from build123d import *

# Parameters (mm, degrees)
SKETCH_1_R          = 9.9
SKETCH_1_R_2        = 1.85
EXTRUDE_1_DEPTH     = 7
SKETCH_2_R          = 12.5
SKETCH_2_R_2        = 1.85
EXTRUDE_2_DEPTH     = 2.5
SKETCH_3_R          = 3.75
EXTRUDE_3_DEPTH     = 6.3
CHAMFER_1_SIZE      = 2
SKETCH_4_R          = 41.5
CUT_EXTRUDE_1_DEPTH = 15.5
EXTRUDE_START       = -0.3
SKETCH_5_R          = 12
SKETCH_5_R_2        = 9.9
EXTRUDE_4_DEPTH     = 0.3


with BuildPart() as part:
    # 草图1 → 凸台-拉伸1 (new body)
    with BuildSketch(Plane(origin=(0, 0, 0), x_dir=(1, 0, 0), z_dir=(0, 1, 0))):
        with Locations(Location((0, 0, 0), (0, 0, 270))):
            Circle(SKETCH_1_R)
        with Locations(Location((6, 0, 0), (0, 0, 270))):
            Circle(SKETCH_1_R_2, mode=Mode.SUBTRACT)
        with Locations(Location((0, -6, 0), (0, 0, 270))):
            Circle(SKETCH_1_R_2, mode=Mode.SUBTRACT)
        with Locations(Location((-6, 0, 0), (0, 0, 270))):
            Circle(SKETCH_1_R_2, mode=Mode.SUBTRACT)
        with Locations(Location((0, 6, 0), (0, 0, 270))):
            Circle(SKETCH_1_R_2, mode=Mode.SUBTRACT)
    extrude(amount=EXTRUDE_1_DEPTH)

    # 草图2 → 凸台-拉伸2 (add)
    with BuildSketch(Plane(origin=(0, 7, 0), x_dir=(1, 0, 0), z_dir=(0, 1, 0))):
        with Locations(Location((0, 0, 0), (0, 0, 270))):
            Circle(SKETCH_2_R)
        with Locations(Location((-6, 0, 0), (0, 0, 270))):
            Circle(SKETCH_2_R_2, mode=Mode.SUBTRACT)
        with Locations(Location((0, -6, 0), (0, 0, 270))):
            Circle(SKETCH_2_R_2, mode=Mode.SUBTRACT)
        with Locations(Location((6, 0, 0), (0, 0, 270))):
            Circle(SKETCH_2_R_2, mode=Mode.SUBTRACT)
        with Locations(Location((0, 6, 0), (0, 0, 270))):
            Circle(SKETCH_2_R_2, mode=Mode.SUBTRACT)
    extrude(amount=EXTRUDE_2_DEPTH)

    # 草图3 → 凸台-拉伸3 (add)
    # profile 1 of 8: a face of its own
    with BuildSketch(Plane(origin=(0, 9.5, 0), x_dir=(1, 0, 0), z_dir=(0, 1, 0))):
        with BuildLine():
            Line((2.25, 0), (-2.25, 0))
            ThreePointArc((-2.25, 0), (-6, -3.75), (-9.75, 0))
            Line((-9.75, 0), (-12.5, 0))
            ThreePointArc((-12.5, 0), (-3.952847075, -11.858541226), (10, -7.5))
            ThreePointArc((10, -7.5), (11.858541226, -3.952847075), (12.5, 0))
            Line((12.5, 0), (9.75, 0))
            ThreePointArc((9.75, 0), (6, -3.75), (2.25, 0))
        make_face()
        with Locations(Location((0, -6, 0), (0, 0, 270))):
            Circle(SKETCH_3_R, mode=Mode.SUBTRACT)
    # profile 2 of 8: a face of its own
    with BuildSketch(Plane(origin=(0, 9.5, 0), x_dir=(1, 0, 0), z_dir=(0, 1, 0))):
        with BuildLine():
            ThreePointArc((-9.75, 0), (-6, 3.75), (-2.25, 0))
            Line((-2.25, 0), (2.25, 0))
            ThreePointArc((2.25, 0), (6, 3.75), (9.75, 0))
            Line((9.75, 0), (12.5, 0))
            ThreePointArc((12.5, 0), (11.858541226, 3.952847075), (10, 7.5))
            ThreePointArc((10, 7.5), (-3.952847075, 11.858541226), (-12.5, 0))
            Line((-12.5, 0), (-9.75, 0))
        make_face()
        with Locations(Location((0, 6, 0), (0, 0, 270))):
            Circle(SKETCH_3_R, mode=Mode.SUBTRACT)
    # profile 3 of 8: a face of its own
    with BuildSketch(Plane(origin=(0, 9.5, 0), x_dir=(1, 0, 0), z_dir=(0, 1, 0))):
        with BuildLine():
            ThreePointArc((10, 7.5), (11.858541226, 3.952847075), (12.5, 0))
            Line((12.5, 0), (25.5, 0))
            ThreePointArc((25.5, 0), (27.696699141, 5.303300859), (33, 7.5))
            Line((33, 7.5), (10, 7.5))
        make_face()
    # profile 4 of 8: a face of its own
    with BuildSketch(Plane(origin=(0, 9.5, 0), x_dir=(1, 0, 0), z_dir=(0, 1, 0))):
        with BuildLine():
            Line((25.5, 0), (12.5, 0))
            ThreePointArc((12.5, 0), (11.858541226, -3.952847075), (10, -7.5))
            Line((10, -7.5), (33, -7.5))
            ThreePointArc((33, -7.5), (27.696699141, -5.303300859), (25.5, 0))
        make_face()
    # profile 5 of 8: a face of its own
    with BuildSketch(Plane(origin=(0, 9.5, 0), x_dir=(1, 0, 0), z_dir=(0, 1, 0))):
        with BuildLine():
            ThreePointArc((33, 7.5), (27.696699141, 5.303300859), (25.5, 0))
            Line((25.5, 0), (28.65, 0))
            ThreePointArc((28.65, 0), (33, 4.35), (37.35, 0))
            Line((37.35, 0), (40.5, 0))
            ThreePointArc((40.5, 0), (38.303300859, 5.303300859), (33, 7.5))
        make_face()
    # profile 6 of 8: a face of its own
    with BuildSketch(Plane(origin=(0, 9.5, 0), x_dir=(1, 0, 0), z_dir=(0, 1, 0))):
        with BuildLine():
            Line((28.65, 0), (25.5, 0))
            ThreePointArc((25.5, 0), (27.696699141, -5.303300859), (33, -7.5))
            ThreePointArc((33, -7.5), (38.303300859, -5.303300859), (40.5, 0))
            Line((40.5, 0), (37.35, 0))
            ThreePointArc((37.35, 0), (33, -4.35), (28.65, 0))
        make_face()
    # profile 7 of 8: a face of its own
    with BuildSketch(Plane(origin=(0, 9.5, 0), x_dir=(1, 0, 0), z_dir=(0, 1, 0))):
        with BuildLine():
            ThreePointArc((33, 7.5), (27.696699141, 5.303300859), (25.5, 0))
            Line((25.5, 0), (28.65, 0))
            ThreePointArc((28.65, 0), (33, 4.35), (37.35, 0))
            Line((37.35, 0), (40.5, 0))
            ThreePointArc((40.5, 0), (38.303300859, 5.303300859), (33, 7.5))
        make_face()
    # profile 8 of 8: a face of its own
    with BuildSketch(Plane(origin=(0, 9.5, 0), x_dir=(1, 0, 0), z_dir=(0, 1, 0))):
        with BuildLine():
            Line((28.65, 0), (25.5, 0))
            ThreePointArc((25.5, 0), (27.696699141, -5.303300859), (33, -7.5))
            ThreePointArc((33, -7.5), (38.303300859, -5.303300859), (40.5, 0))
            Line((40.5, 0), (37.35, 0))
            ThreePointArc((37.35, 0), (33, -4.35), (28.65, 0))
        make_face()
    extrude(amount=EXTRUDE_3_DEPTH)

    # 倒角1
    # the kernel refuses this chamfer: 2 mm, written as the material it adds along each edge
    with BuildSketch(Plane(origin=(0, 9.5, 6), x_dir=(0, 0, 1), z_dir=(-1, 0, 0))) as chamfer_1_piece_1_section:
        Polygon((3.75 - CHAMFER_1_SIZE, 0), (3.75, CHAMFER_1_SIZE), (3.75, 0), align=None)
    chamfer_1_piece_1 = revolve(axis=Axis((0, 9.5, 6), (0, 1, 0)), mode=Mode.PRIVATE)
    chamfer_1_piece_1 = chamfer_1_piece_1 - Plane(origin=(0, 10.553600351, 6), x_dir=(0, 0, 1), z_dir=(0, -1, 0)) * Cylinder(1.85, 15, mode=Mode.PRIVATE)
    add(chamfer_1_piece_1)
    with BuildSketch(Plane(origin=(-6, 9.5, 0), x_dir=(-1, 0, 0), z_dir=(0, 0, 1))) as chamfer_1_piece_2_section:
        Polygon((3.75 - CHAMFER_1_SIZE, 0), (3.75, -CHAMFER_1_SIZE), (3.75, 0), align=None)
    chamfer_1_piece_2 = revolve(axis=Axis((-6, 9.5, 0), (0, -1, 0)), mode=Mode.PRIVATE)
    chamfer_1_piece_2 = chamfer_1_piece_2 - Plane(origin=(-6, 10.553600351, 0), x_dir=(0, 0, 1), z_dir=(0, -1, 0)) * Cylinder(1.85, 15, mode=Mode.PRIVATE)
    add(chamfer_1_piece_2)
    with BuildSketch(Plane(origin=(0, 9.5, -6), x_dir=(0, 0, 1), z_dir=(-1, 0, 0))) as chamfer_1_piece_3_section:
        Polygon((3.75 - CHAMFER_1_SIZE, 0), (3.75, CHAMFER_1_SIZE), (3.75, 0), align=None)
    chamfer_1_piece_3 = revolve(axis=Axis((0, 9.5, -6), (0, 1, 0)), mode=Mode.PRIVATE)
    chamfer_1_piece_3 = chamfer_1_piece_3 - Plane(origin=(0, 10.553600351, -6), x_dir=(0, 0, 1), z_dir=(0, -1, 0)) * Cylinder(1.85, 16, mode=Mode.PRIVATE)
    add(chamfer_1_piece_3)
    with BuildSketch(Plane(origin=(6, 9.5, 0), x_dir=(1, 0, 0), z_dir=(0, 0, -1))) as chamfer_1_piece_4_section:
        Polygon((3.75 - CHAMFER_1_SIZE, 0), (3.75, -CHAMFER_1_SIZE), (3.75, 0), align=None)
    chamfer_1_piece_4 = revolve(axis=Axis((6, 9.5, 0), (0, -1, 0)), mode=Mode.PRIVATE)
    chamfer_1_piece_4 = chamfer_1_piece_4 - Plane(origin=(6, 10.553600351, 0), x_dir=(0, 0, 1), z_dir=(0, -1, 0)) * Cylinder(1.85, 15, mode=Mode.PRIVATE)
    add(chamfer_1_piece_4)

    # 草图4 → 切除-拉伸1 (cut)
    with BuildSketch(Plane(origin=(0, 15.8, 0), x_dir=(1, 0, 0), z_dir=(0, 1, 0))):
        Circle(SKETCH_4_R)
    extrude(amount=-CUT_EXTRUDE_1_DEPTH, mode=Mode.SUBTRACT)

    # 草图5 → 凸台-拉伸4 (add)
    with BuildSketch(Plane(origin=(0, 0.3, 0), x_dir=(1, 0, 0), z_dir=(0, 1, 0)).offset(EXTRUDE_START)):
        with Locations(Location((0, 0, 0), (0, 0, 270))):
            Circle(SKETCH_5_R)
        Circle(SKETCH_5_R_2, mode=Mode.SUBTRACT)
    extrude(amount=EXTRUDE_4_DEPTH)


solid = part.part
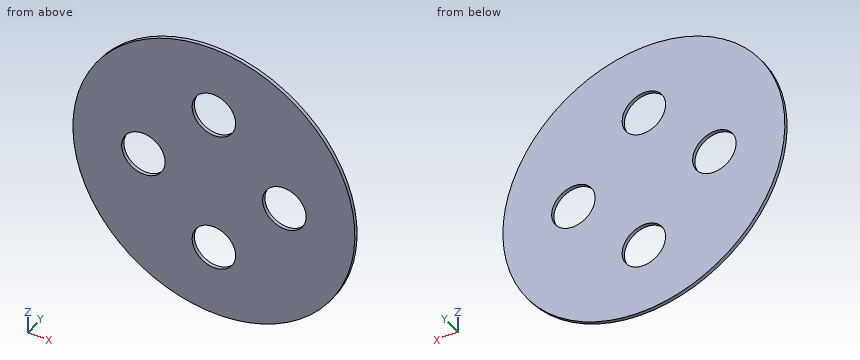
The model under review builds one solid part; all positions refer to its coordinate system, in mm. Round coordinates to 2 decimals unless told otherwise and drop trailing zeros. Write each loop counter-clockwise with the first axis right and the second up, starting at its lowest first coordinate (ties: lowest second). Pieces come first, ordered by that corner, then holes. Notation, with made-up numbers: M 40,43 L 46,43 A22 cw 46,74 Z; hole C 27.25,38.25 d6. An arc over 180 degrees is marked long. Use a Markdown table: item, result. Add a question column.
Q1. We need section C-C, the plane x = 6. State the section outline as (y, z) points, plus the area to 3 significant figures.
Q2. We need section B-B, the plane y = 0.2. State the section outline as (x, z) points, plus the area to 3 significant figures.
Q3. To check wall thickness, follow line 1 (X direction, y = 0.15, z = 0); line 2 (X direction, y = 0.15, z = -4.5); line 3 (Z direction, x = -6, y = 0.25). State the ranges of each line that lie inside material, in increasing order.
Q4. Insertion check: pin 1 (3.5 mm diameter, centred on x = 0, z = -6, fed in from +Y); pin 2 (4.5 mm diameter, centred on x = 6, z = 0, fed in from -Y). Each pin has a flat end and moves straight along its axis. Give the tip position at first contact, or say it passes through.
Q5. We need section D-D, the plane z = 6. State the section outline as (x, y) points, plus the area to 3 significant figures.
Q6. We need section A-A, the plane z = 0. State the section outline as (x, y) points, plus the area to 3 significant figures.
Findings below:
| question | item | result |
|---|---|---|
| 1 | outline | M 0,-10.39 L 0.3,-10.39 L 0.3,-1.85 L 0,-1.85 Z; M 0,1.85 L 0.3,1.85 L 0.3,10.39 L 0,10.39 Z |
| 1 | area | 5.13 mm² |
| 2 | outline | C 0,0 d24; hole C -6,0 d3.7; hole C 0,-6 d3.7; hole C 0,6 d3.7; hole C 6,0 d3.7 |
| 2 | area | 409 mm² |
| 3 | line 1 | x = -12 to -7.85, -4.15 to 4.15, 7.85 to 12 |
| 3 | line 2 | x = -11.12 to -1.08, 1.08 to 11.12 |
| 3 | line 3 | z = -10.39 to -1.85, 1.85 to 10.39 |
| 4 | pin 1 | passes through |
| 4 | pin 2 | stops at y = 0 |
| 5 | outline | M -10.39,0 L -1.85,0 L -1.85,0.3 L -10.39,0.3 Z; M 1.85,0 L 10.39,0 L 10.39,0.3 L 1.85,0.3 Z |
| 5 | area | 5.13 mm² |
| 6 | outline | M -12,0 L -7.85,0 L -7.85,0.3 L -12,0.3 Z; M -4.15,0 L 4.15,0 L 4.15,0.3 L -4.15,0.3 Z; M 7.85,0 L 12,0 L 12,0.3 L 7.85,0.3 Z |
| 6 | area | 4.98 mm² |
